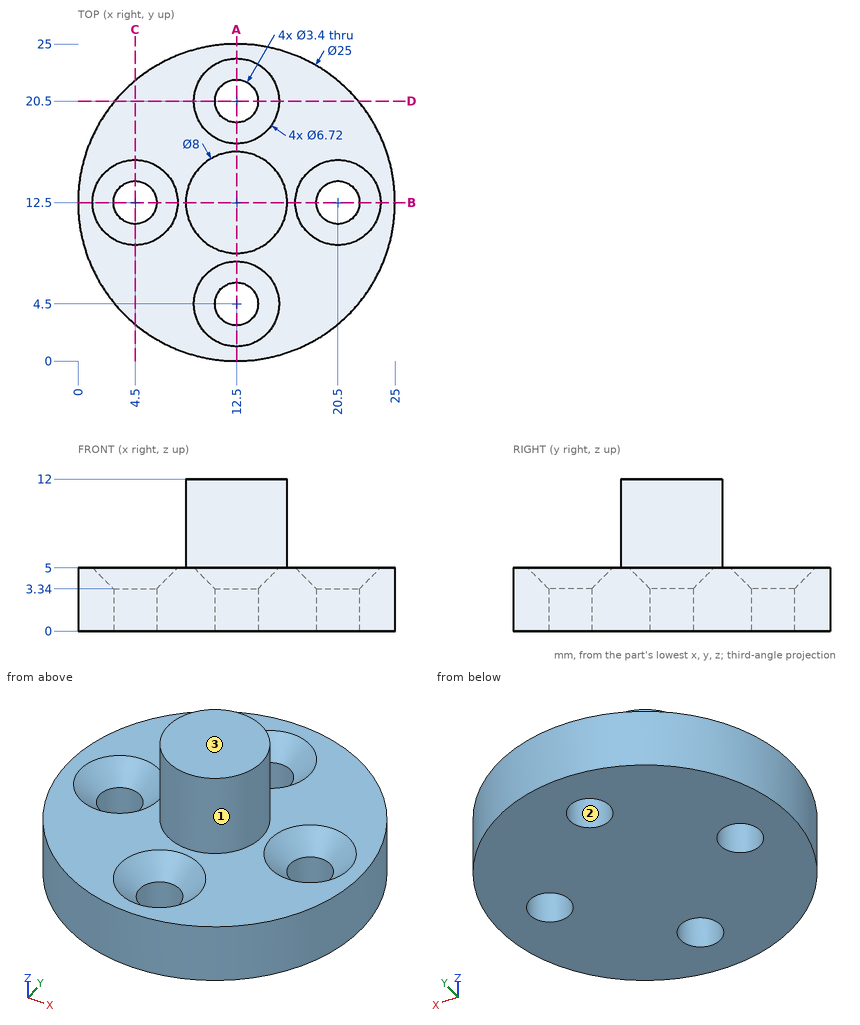
Geometry check sheet. Reference: drawing and pictorial views, mm from the part's lowest x, y, z. Round coordinates to 2 decimals unless told otherwise and drop trailing zeros. Loops run counter-clockwise (first coordinate to the right, second up) from the corner with the lowest first, then second, coordinate; pieces in that order, holes last.
1. Scan lines: probe 1 along Y at (x, z) = (12.5, 1.75); probe 2 along Z at (x, y) = (9.5, 7.25); probe 3 along X at (y, z) = (20.5, 4). Record each from-to range of solid material in increasing order.
2. Sectioned sample at C-C on x = 4.5. Record the boundary of the cut face in (y, z).
3. Sectioned sample at A-A on x = 12.5. Record the boundary of the cut face in (y, z).
4. Gauge pin test, flat ends, axial feed: pin 1 Ø4.5 at (x, y) = (20.5, 12.5) entering from -Z; pin 2 Ø4 at (y, z) = (5.5, 5.5) entering from -X; pin 3 Ø3 at (x, y) = (12.5, 4.5) entering from +Z; pin 4 Ø5.5 at (x, y) = (12.5, 20.5) entering from +Z. Record the tip position at first contact, or that the pin passes through.
5. Mould release check, pull along X, two halves, no side actions. Record for the marked faces 1, 2 and 3: released by +X, released by -X, zero draft, split by the parting line, or undercut.
Recorded:
1. probe 1: y = 0 to 2.8, 6.2 to 18.8, 22.2 to 25
1. probe 2: z = 0 to 5
1. probe 3: x = 2.9 to 10.14, 14.86 to 22.1
2. outline: (2.9, 0) - (10.8, 0) - (10.8, 3.34) - (9.14, 5) - (2.9, 5) - close; (14.2, 0) - (22.1, 0) - (22.1, 5) - (15.86, 5) - (14.2, 3.34) - close
3. outline: (0, 0) - (2.8, 0) - (2.8, 3.34) - (1.14, 5) - (0, 5) - close; (6.2, 0) - (18.8, 0) - (18.8, 3.34) - (17.14, 5) - (16.5, 5) - (16.5, 12) - (8.5, 12) - (8.5, 5) - (7.86, 5) - (6.2, 3.34) - close; (22.2, 0) - (25, 0) - (25, 5) - (23.86, 5) - (22.2, 3.34) - close
4. pin 1: stops at z = 0
4. pin 2: stops at x = 1.07
4. pin 3: passes through
4. pin 4: stops at z = 4.39
5. face 1: split by the parting line
5. face 2: undercut
5. face 3: zero draft
